The model under review builds one solid part; all positions refer to its coordinate system, in mm. A direction names the side the tool comes from. Coordinates: 2 decimals unless noted, no trailing zeros. Loops run counter-clockwise (first coordinate to the right, second up) from the corner with the lowest first, then second, coordinate; pieces in that order, holes last. Notation, with made-up numbers: (14, 36.5) - (28, 36.5) arc R9 ccw to (28, 42.5) - close; hole circle Ø3 at (69.5, -7.5). An arc over 180 degrees is marked (long way). Use a Markdown table: item, result. Add a question column.
1) Add section C-C, the plane y = -9. Give the boundary of the cut face in (x, z).
2) To check wall thickness, follow L1, parallel to X at y = -15, z = 2; L2, parallel to X at y = -12.5, z = -3.75; L3, parallel to Y at x = -11, z = -0.25. State the ranges of each line that lie inside material, in increasing order. Write a range as [from, to].
3) Add section B-B, the plane x = -1.5. Give the boundary of the cut face in (y, z), and give its area (3 significant figures).
4) The part is to be moulded in two halves that separate along Y. For faces 1 (the cylindrical face through (12.718, 12.738, -0.07)), 2 (the cylindrical face through (4.383, -15.158, 0.07)), 3 (the cylindrical face through (7.51, 11.22, 0.07)), say which applies: pulls with the +Y half, pulls with the -Y half, needs draft (parallel to the pull), parting line crosses it, or undercut.
5) For faces 4 (the cylindrical face through (13.242, 2.625, 0.07)), 5 (the cylindrical face through (-13.24, 2.64, 0.07)), 6 (the flat face through (0, 2, 0)), list the 3-axis set-ups (+Z, -Z, +X, -X, +Y, -Y) from which the entire face can be reached by the end or side of a thin tool; tool diameter is ignored.
6) Add section D-D, the plane x = -9.5. Give the boundary of the cut face in (y, z), and give its area (3 significant figures).
7) Clearance check with flat-ended pins moving along their axes: pin 1 (2 mm diameter, centred on x = -14.5, y = -9, fed in from -Z); pin 2 (6 mm diameter, centred on y = 3.5, z = 3, fed in from +X); pin 3 (1.5 mm diameter, centred on y = 5, z = -2, fed in from +X); pin 4 (2 mm diameter, centred on x = 11.5, z = 2.5, fed in from -Y). State where each tip first meets the part, or that it passes through.
8) Add section A-A, the plane x = 15.5. Give the boundary of the cut face in (y, z).
Autodesk Inventor part; units mm, degrees
ref_plane "YZ Plane" through (0, 0, 0) normal (1, 0, 0) x (0, 1, 0)
ref_plane "XZ Plane" through (0, 0, 0) normal (0, 1, 0) x (-1, 0, 0)
ref_plane "XY Plane" through (0, 0, 0) normal (0, 0, 1) x (1, 0, 0)
sketch "스케치1" plane through (0, 0, 0) normal (0, 0, 1) x (1, 0, 0)
  circle A0 centre (0, 0) radius 18
  dimension "d0" = 36
extrude "돌출1" add sketch "스케치1" along normal mid plane 10
sketch "스케치2" plane through (0, 0, 5) normal (0, 0, 1) x (1, 0, 0)
  circle A0 centre (0, 0) radius 18
  circle A1 centre (0, 0) radius 13.5
  line L0 (0, 0) -> (0, 22.2867) construction
  line L1 (-1, 0) -> (-1, 22.2867) construction
  line L2 (-2, 0) -> (-2, 22.2867) construction
  arc A2 (-1, 17.9722) -> (-2, 13.351) centre (9.3, 13.3246) ccw
  arc A3 (2, 13.351) -> (1, 17.9722) centre (-9.3, 13.3246) ccw
  point P0 (1, 17.9722)
  point P1 (2, 13.351)
  dimension "d3" = 4.5
  dimension "d4" = 1
  dimension "d5" = 1
  dimension "d6" = 11.3
extrude "돌출2" cut sketch "스케치2" against normal blind 15 contours A0 A2 A1 A3 picked at (16.1915, -2.5264)
pattern_circular "원형 패턴1" count 16 over 360 about axis through (0, 0, 5) along (0, 0, -1)
sketch "스케치3" plane through (0, 0, 5) normal (0, 0, 1) x (1, 0, 0)
  arc A0 (2, 13.351) -> (1, 17.9722) centre (-9.3, 13.3246) ccw
  arc A1 (1, 17.9722) -> (-1, 17.9722) centre (0, 0) ccw
  arc A2 (-1, 17.9722) -> (-2, 13.351) centre (9.3, 13.3246) ccw
  arc A3 (-2, 13.351) -> (-3.2615, 13.1001) centre (0, 0) ccw
  arc A4 (-3.2615, 13.1001) -> (-5.9538, 16.9868) centre (-13.6911, 8.7513) ccw
  arc A5 (-5.9538, 16.9868) -> (-7.8015, 16.2215) centre (0, 0) ccw
  arc A6 (-7.8015, 16.2215) -> (-6.957, 11.5694) centre (3.493, 15.8692) ccw
  arc A7 (-6.957, 11.5694) -> (-8.0264, 10.8548) centre (0, 0) ccw
  arc A8 (-8.0264, 10.8548) -> (-12.0012, 13.4154) centre (-15.998, 2.8458) ccw
  arc A9 (-12.0012, 13.4154) -> (-13.4154, 12.0012) centre (0, 0) ccw
  arc A10 (-13.4154, 12.0012) -> (-10.8548, 8.0264) centre (-2.8458, 15.998) ccw
  arc A11 (-10.8548, 8.0264) -> (-11.5694, 6.957) centre (0, 0) ccw
  arc A12 (-11.5694, 6.957) -> (-16.2215, 7.8015) centre (-15.8692, -3.493) ccw
  arc A13 (-16.2215, 7.8015) -> (-16.9868, 5.9538) centre (0, 0) ccw
  arc A14 (-16.9868, 5.9538) -> (-13.1001, 3.2615) centre (-8.7513, 13.6911) ccw
  arc A15 (-13.1001, 3.2615) -> (-13.351, 2) centre (0, 0) ccw
  arc A16 (-13.351, 2) -> (-17.9722, 1) centre (-13.3246, -9.3) ccw
  arc A17 (-17.9722, 1) -> (-17.9722, -1) centre (0, 0) ccw
  arc A18 (-17.9722, -1) -> (-13.351, -2) centre (-13.3246, 9.3) ccw
  arc A19 (-13.351, -2) -> (-13.1001, -3.2615) centre (0, 0) ccw
  arc A20 (-13.1001, -3.2615) -> (-16.9868, -5.9538) centre (-8.7513, -13.6911) ccw
  arc A21 (-16.9868, -5.9538) -> (-16.2215, -7.8015) centre (0, 0) ccw
  arc A22 (-16.2215, -7.8015) -> (-11.5694, -6.957) centre (-15.8692, 3.493) ccw
  arc A23 (-11.5694, -6.957) -> (-10.8548, -8.0264) centre (0, 0) ccw
  arc A24 (-10.8548, -8.0264) -> (-13.4154, -12.0012) centre (-2.8458, -15.998) ccw
  arc A25 (-13.4154, -12.0012) -> (-12.0012, -13.4154) centre (0, 0) ccw
  arc A26 (-12.0012, -13.4154) -> (-8.0264, -10.8548) centre (-15.998, -2.8458) ccw
  arc A27 (-8.0264, -10.8548) -> (-6.957, -11.5694) centre (0, 0) ccw
  arc A28 (-6.957, -11.5694) -> (-7.8015, -16.2215) centre (3.493, -15.8692) ccw
  arc A29 (-7.8015, -16.2215) -> (-5.9538, -16.9868) centre (0, 0) ccw
  arc A30 (-5.9538, -16.9868) -> (-3.2615, -13.1001) centre (-13.6911, -8.7513) ccw
  arc A31 (-3.2615, -13.1001) -> (-2, -13.351) centre (0, 0) ccw
  arc A32 (-2, -13.351) -> (-1, -17.9722) centre (9.3, -13.3246) ccw
  arc A33 (-1, -17.9722) -> (1, -17.9722) centre (0, 0) ccw
  arc A34 (1, -17.9722) -> (2, -13.351) centre (-9.3, -13.3246) ccw
  arc A35 (2, -13.351) -> (3.2615, -13.1001) centre (0, 0) ccw
  arc A36 (3.2615, -13.1001) -> (5.9538, -16.9868) centre (13.6911, -8.7513) ccw
  arc A37 (5.9538, -16.9868) -> (7.8015, -16.2215) centre (0, 0) ccw
  arc A38 (7.8015, -16.2215) -> (6.957, -11.5694) centre (-3.493, -15.8692) ccw
  arc A39 (6.957, -11.5694) -> (8.0264, -10.8548) centre (0, 0) ccw
  arc A40 (8.0264, -10.8548) -> (12.0012, -13.4154) centre (15.998, -2.8458) ccw
  arc A41 (12.0012, -13.4154) -> (13.4154, -12.0012) centre (0, 0) ccw
  arc A42 (13.4154, -12.0012) -> (10.8548, -8.0264) centre (2.8458, -15.998) ccw
  arc A43 (10.8548, -8.0264) -> (11.5694, -6.957) centre (0, 0) ccw
  arc A44 (11.5694, -6.957) -> (16.2215, -7.8015) centre (15.8692, 3.493) ccw
  arc A45 (16.2215, -7.8015) -> (16.9868, -5.9538) centre (0, 0) ccw
  arc A46 (16.9868, -5.9538) -> (13.1001, -3.2615) centre (8.7513, -13.6911) ccw
  arc A47 (13.1001, -3.2615) -> (13.351, -2) centre (0, 0) ccw
  arc A48 (13.351, -2) -> (17.9722, -1) centre (13.3246, 9.3) ccw
  arc A49 (17.9722, -1) -> (17.9722, 1) centre (0, 0) ccw
  arc A50 (17.9722, 1) -> (13.351, 2) centre (13.3246, -9.3) ccw
  arc A51 (13.351, 2) -> (13.1001, 3.2615) centre (0, 0) ccw
  arc A52 (13.1001, 3.2615) -> (16.9868, 5.9538) centre (8.7513, 13.6911) ccw
  arc A53 (16.9868, 5.9538) -> (16.2215, 7.8015) centre (0, 0) ccw
  arc A54 (16.2215, 7.8015) -> (11.5694, 6.957) centre (15.8692, -3.493) ccw
  arc A55 (11.5694, 6.957) -> (10.8548, 8.0264) centre (0, 0) ccw
  arc A56 (10.8548, 8.0264) -> (13.4154, 12.0012) centre (2.8458, 15.998) ccw
  arc A57 (13.4154, 12.0012) -> (12.0012, 13.4154) centre (0, 0) ccw
  arc A58 (12.0012, 13.4154) -> (8.0264, 10.8548) centre (15.998, 2.8458) ccw
  arc A59 (8.0264, 10.8548) -> (6.957, 11.5694) centre (0, 0) ccw
  arc A60 (6.957, 11.5694) -> (7.8015, 16.2215) centre (-3.493, 15.8692) ccw
  arc A61 (7.8015, 16.2215) -> (5.9538, 16.9868) centre (0, 0) ccw
  arc A62 (5.9538, 16.9868) -> (3.2615, 13.1001) centre (13.6911, 8.7513) ccw
  arc A63 (3.2615, 13.1001) -> (2, 13.351) centre (0, 0) ccw
  line L0 (-4.0823, 0) -> (5.9538, 0) construction
  line L1 (-2.2361, 2) -> (2.2361, 2)
  line L2 (-2.2361, -2) -> (2.2361, -2)
  arc A64 (-2.2361, 2) -> (-2.2361, -2) centre (0, 0) ccw
  arc A65 (2.2361, -2) -> (2.2361, 2) centre (0, 0) ccw
  point P0 (3, 0)
  point P1 (-3, 0)
  dimension "d13" = 2
  dimension "d14" = 2
  dimension "d15" = 6
extrude "돌출3" cut sketch "스케치3" against normal through all contours L1 A65 L2 A64
properties part number "피니언"
From the geometry:
| question | item | result |
|---|---|---|
| 1 | outline | (-11.72, -5) - (11.72, -5) - (11.72, 5) - (-11.72, 5) - close |
| 2 | L1 | x = [-7.77, -4.28], [-1.88, 1.88], [4.28, 7.77] |
| 2 | L2 | x = [-12.95, -10.13], [-7.29, 7.29], [10.13, 12.95] |
| 2 | L3 | y = [-12.98, -8.17], [-7.83, 7.83], [8.17, 12.98] |
| 3 | outline | (-16.65, -5) - (-2, -5) - (-2, 5) - (-16.65, 5) - close; (2, -5) - (16.65, -5) - (16.65, 5) - (2, 5) - close |
| 3 | area | 293 mm^2 |
| 4 | face 1 | pulls with the +Y half |
| 4 | face 2 | pulls with the -Y half |
| 4 | face 3 | undercut |
| 5 | face 4 | +Z, -Z, +X |
| 5 | face 5 | +Z, -Z, -X |
| 5 | face 6 | +Z, -Z |
| 6 | outline | (-12.09, -5) - (12.09, -5) - (12.09, 5) - (-12.09, 5) - close |
| 6 | area | 242 mm^2 |
| 7 | pin 1 | passes through |
| 7 | pin 2 | stops at x = 17.99 |
| 7 | pin 3 | stops at x = 16.79 |
| 7 | pin 4 | stops at y = -13.42 |
| 8 | outline | (-7.8, -5) - (-4.63, -5) - (-4.63, 5) - (-7.8, 5) - close; (-1.79, -5) - (1.79, -5) - (1.79, 5) - (-1.79, 5) - close; (4.63, -5) - (7.8, -5) - (7.8, 5) - (4.63, 5) - close |
